Geometry: final body of the model. Coordinates: model frame, mm. A direction names the side the tool comes from. Give positions to 0.01 mm unless a question says otherwise; leave off trailing zeros. Loops run counter-clockwise (first coordinate to the right, second up) from the corner with the lowest first, then second, coordinate; pieces in that order, holes last.
from build123d import *

# Parameters (mm, degrees)
F0_W     = 10
F0_H     = 5
F0_H_2   = 44.692295
F0_H_3   = 45.307705
F0_H_4   = 45.157636
F0_H_5   = 44.842364
F1_DEPTH = 1000


with BuildPart() as f1:
    # F0 (on Front) → F1 (new body)
    with BuildSketch(Plane.XZ):
        Polygon((40.000761, 0), (0, 0), (-40.000761, 0), (-40.000761, -5), (0, -5), (40.000761, -5), align=None)
        Polygon((-40.000761, 0), (0, 0), (40.000761, 0), (40.000761, 5), (0, 5), (-40.000761, 5), align=None)
        with Locations((-45.000761, -2.5)):
            Rectangle(F0_W, F0_H)
        with Locations((-45.000761, 2.5)):
            Rectangle(F0_W, F0_H)
        with Locations((45.000761, 2.5)):
            Rectangle(F0_W, F0_H)
        with Locations((45.000761, -2.5)):
            Rectangle(F0_W, F0_H)
        with Locations((-45.000761, -27.346147)):
            Rectangle(F0_W, F0_H_2)
        with Locations((-45.000761, 27.653852)):
            Rectangle(F0_W, F0_H_3)
        with Locations((45.000761, -27.578818)):
            Rectangle(F0_W, F0_H_4)
        with Locations((45.000761, 27.421182)):
            Rectangle(F0_W, F0_H_5)
    extrude(amount=F1_DEPTH)


solid = f1.part
Item 1: Section query C-C on x = 12. Return loops of the section in (y, z).
Values follow:
outline: (-1000, -5) - (0, -5) - (0, 5) - (-1000, 5) - close
Item 2: Ray query, probe 1 along X at (y, z) = (-806, -38); probe 2 along Z at (x, y) = (30, -812). Return the intervals inside material, ascending.
Values follow:
probe 1: x = -50 to -40, 40 to 50
probe 2: z = -5 to 5
Item 3: Pin query (flat end, axial travel): pin 1 (24 mm diameter, centred on x = 19.5, y = -526.5, fed in from -Z); pin 2 (1.5 mm diameter, centred on x = -13.5, y = -342.5, fed in from +Z); pin 3 (5 mm diameter, centred on x = 47.5, y = -519, fed in from +Z). Return the tip coordinate at first contact, or that it passes through.
Values follow:
pin 1: stops at z = -5
pin 2: stops at z = 5
pin 3: stops at z = 49.84
Item 4: Draft query along X for faces 1 (the face through (-50.001, -493, 1)), 2 (the face through (3, 0, 0)), 3 (the face through (-1, -493, -5)). Return one class per face: +X half, -X half, draft (parallel to the pull), parting line (faces both ways), or undercut.
Values follow:
face 1: -X half
face 2: draft
face 3: undercut
Item 5: Set-up query: faces 4 (the face through (40.001, -493, -28)), 5 (the face through (1, -493, 5)), 6 (the face through (3, -1000, 0)). Return all of +Z, -Z, +X, -X, +Y, -Y with unobstructed straight access to the full face (end or side cutting, diameter ignored); none if empty.
Values follow:
face 4: -Z, +Y, -Y
face 5: +Z, +Y, -Y
face 6: +Z, -Z, +X, -X, -Y
Item 6: Section query B-B on y = -896. Return loops of the section in (x, z).
Values follow:
outline: (-50, -49.69) - (-40, -49.69) - (-40, -5) - (40, -5) - (40, -50.16) - (50, -50.16) - (50, 49.84) - (40, 49.84) - (40, 5) - (-40, 5) - (-40, 50.31) - (-50, 50.31) - close
Item 7: Section query A-A on z = -27. Return loops of the section in (x, y), plus the area to 3 significant figures.
Values follow:
outline: (-50, -1000) - (-40, -1000) - (-40, 0) - (-50, 0) - close; (40, -1000) - (50, -1000) - (50, 0) - (40, 0) - close
area: 20,000 mm2
